Model file for the job. Use its own axes, mm. Face numbers are marked on the shaded views. Round coordinates to 2 decimals unless told otherwise and drop trailing zeros. Order: outer loops, then holes, each group sorted by start corner. A loop starts at its lowest first (then second) coordinate and runs counter-clockwise, first axis right, second up. Notation, with made-up numbers: (-25, -14) - (-1, -14) arc R22 ccw to (-1, 8) - close; hole circle Ø8 at (-39.5, -36). An arc over 180 degrees is marked (long way). Put each result on its own line as item: value. Start each with the question number.
Item 1: Pin check, flat tips, straight feed: pin 1 Ø6 at (x, z) = (-21.63, 12.4) entering from +Y; pin 2 Ø12 at (x, z) = (-6, 9.5) entering from -Y; pin 3 Ø10.5 at (x, z) = (-9.63, 12.4) entering from -Y; pin 4 Ø7 at (x, y) = (-32.87, -8) entering from +Z. Stop position of each tip, or through.
Item 2: Saw through at D-D on y = -5.75. State how many separate pieces and enclosed holes the cut face has, plus the area to 3 significant figures.
Item 3: Saw through at B-B on y = 3. List the corners of the cut face in (x, z), plus the area to 3 significant figures.
Item 4: Saw through at C-C on z = 2.25. List the corners of the cut face in (x, y), plus the area to 3 significant figures.
Item 5: Probe probe 1 along X at (y, z) = (-10.25, 4.25); probe 2 along Y at (x, z) = (-33.5, 16); probe 3 along Z at (x, y) = (-16, -12.25). List the from-to ranges inside material, lowest first.
Item 6: Saw through at A-A on z = 12.4. List the corners of the cut face in (x, y), plus the area to 3 significant figures.
Item 7: Mould opens along Z. For the marked faces 1, 2 and 3 say: pulls with the +Z half, pulls with the -Z half, needs draft (parallel to the pull), parting line crosses it, or undercut.
```python
from build123d import *

# Parameters (mm, degrees)
F0_W     = 55
F0_H     = 18
F0_R     = 3
F0_R_2   = 3.1
F0_R_3   = 3.2
F0_R_4   = 3.3
F1_DEPTH = 4.8
F0_H_2   = 7.2
F2_DEPTH = 20
F3_R     = 3
F3_R_2   = 3.1
F3_R_3   = 3.2
F3_R_4   = 3.3
F4_DEPTH = 25
F5_SIZE  = 0.8


with BuildPart() as f1:
    # F0 (on Top) → F1 (new body)
    with BuildSketch(Plane.XY):
        with Locations((-27.5, -8.003877)):
            Rectangle(F0_W, F0_H)
        with Locations((-44.867948, -8.003877)):
            Circle(F0_R, mode=Mode.SUBTRACT)
        with Locations((-32.867948, -8.003877)):
            Circle(F0_R_2, mode=Mode.SUBTRACT)
        with Locations((-20.867948, -8.003877)):
            Circle(F0_R_3, mode=Mode.SUBTRACT)
        with Locations((-8.867948, -8.003877)):
            Circle(F0_R_4, mode=Mode.SUBTRACT)
    extrude(amount=F1_DEPTH)

    # F0 (on Top) → F2 (join)
    with BuildSketch(Plane.XY):
        with Locations((-27.5, 4.596123)):
            Rectangle(F0_W, F0_H_2)
    extrude(amount=F2_DEPTH)

    # F3 (on face) → F4 (cut)
    with BuildSketch(Plane.XZ.offset(-0.996123)):
        with Locations((-45.631237, 12.4)):
            Circle(F3_R)
        with Locations((-33.631237, 12.4)):
            Circle(F3_R_2)
        with Locations((-21.631237, 12.4)):
            Circle(F3_R_3)
        with Locations((-9.631237, 12.4)):
            Circle(F3_R_4)
    extrude(amount=-F4_DEPTH, mode=Mode.SUBTRACT)

    # F5
    f5_edges = [f1.edges().sort_by_distance(p)[0] for p in [
        (-47.867948, -8.003877, 0),
        (-35.967948, -8.003877, 0),
        (-24.067948, -8.003877, 0),
        (-12.167948, -8.003877, 0),
    ]]
    chamfer(f5_edges, length=F5_SIZE)


solid = f1.part
```
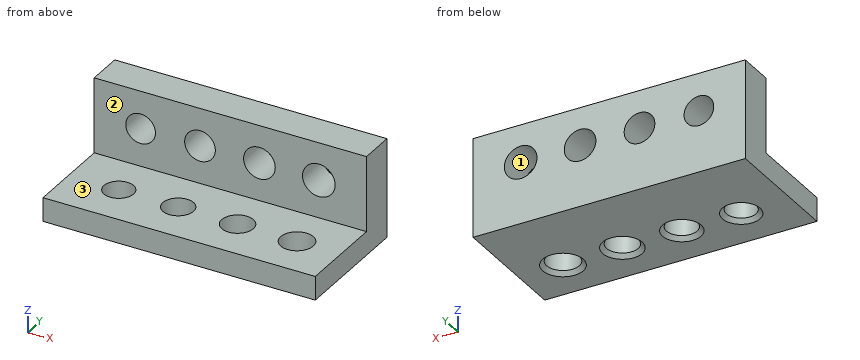
Results found:
1. pin 1: passes through
1. pin 2: stops at y = -17
1. pin 3: stops at y = 1
1. pin 4: stops at z = 4.8
2. separate pieces: 5
2. enclosed holes: 0
2. area: 176 mm²
3. outline: (-55, 0) - (0, 0) - (0, 20) - (-55, 20) - close; hole circle Ø6 at (-45.63, 12.4); hole circle Ø6.2 at (-33.63, 12.4); hole circle Ø6.4 at (-21.63, 12.4); hole circle Ø6.6 at (-9.63, 12.4)
3. area: 975 mm²
4. outline: (-55, -17) - (0, -17) - (0, 8.2) - (-55, 8.2) - close; hole circle Ø6 at (-44.87, -8); hole circle Ø6.2 at (-32.87, -8); hole circle Ø6.4 at (-20.87, -8); hole circle Ø6.6 at (-8.87, -8)
4. area: 1,260 mm²
5. probe 1: x = -55 to -46.86, -42.88 to -35, -30.73 to -23.15, -18.59 to -11.29, -6.45 to 0
5. probe 2: y = 1 to 8.2
5. probe 3: z = 0 to 4.8
6. outline: (-55, 1) - (-48.63, 1) - (-48.63, 8.2) - (-55, 8.2) - close; (-42.63, 1) - (-36.73, 1) - (-36.73, 8.2) - (-42.63, 8.2) - close; (-30.53, 1) - (-24.83, 1) - (-24.83, 8.2) - (-30.53, 8.2) - close; (-18.43, 1) - (-12.93, 1) - (-12.93, 8.2) - (-18.43, 8.2) - close; (-6.33, 1) - (0, 1) - (0, 8.2) - (-6.33, 8.2) - close
6. area: 215 mm²
7. face 1: undercut
7. face 2: needs draft
7. face 3: pulls with the +Z half
